Source: CAD feature listing. Evaluate the final solid. Frame: model axes, mm. Round coordinates to 2 decimals unless told otherwise and drop trailing zeros. Loops run counter-clockwise (first coordinate to the right, second up) from the corner with the lowest first, then second, coordinate; pieces in that order, holes last.
(1) Section D-D, the plane y = 15.5. Return the cut outline in (x, z).
(2) Section C-C, the plane z = -12. Return the cut outline in (x, y), plus the area to 3 significant figures.
(3) Section B-B, the plane y = -10. Return the cut outline in (x, z), plus the area to 3 significant figures.
(4) Material intervals for probe 1 along Y at (x, z) = (0, -24.5); probe 2 along Y at (x, z) = (0, -1.3), sorted ascending.
(5) Section A-A, the plane x = 0. Return the cut outline in (y, z).
(6) First-contact query: pin 1 Ø1 at (y, z) = (-12, -12.5) entering from +X; pin 2 Ø12 at (x, z) = (-2.5, -11.5) entering from -Y; pin 3 Ø2 at (x, z) = (-14, -4.5) entering from -Y. Flat tips, straight axial feed; report the tip coordinate or a pass-through.
(7) Mould query, pull axis Y, two halves, no side actions, for faces 1 (the flat face through (6, 20, -30)), 2 (the flat face through (-8, -11, -5)), 3 (the cylindrical face through (-2.343, -17.847, -18.311)), 4 (the cylindrical face through (-4.336, 19.524, -14.79)). Classes: pulls with the +Y half, pulls with the -Y half, needs draft (parallel to the pull), parting line crosses it, or undercut.
```python
from build123d import *

# Parameters (mm, degrees)
F0_R     = 20
F0_R_2   = 13.25
F1_DEPTH = 5
F2_R     = 20
F2_R_2   = 18
F3_DEPTH = 25
F4_R     = 30
F4_R_2   = 18
F5_DEPTH = 2


with BuildPart() as f1:
    # F0 (on Top) → F1 (new body)
    with BuildSketch(Plane.XY):
        Circle(F0_R)
        Circle(F0_R_2, mode=Mode.SUBTRACT)
    extrude(amount=-F1_DEPTH)

    # F2 (on face) → F3 (join)
    with BuildSketch(Plane(origin=(0, 0, -5), x_dir=(1, 0, 0), z_dir=(0, 0, -1))):
        Circle(F2_R)
        Circle(F2_R_2, mode=Mode.SUBTRACT)
    extrude(amount=F3_DEPTH)

    # F4 (on face) → F5 (join)
    with BuildSketch(Plane(origin=(0, 0, -30), x_dir=(1, 0, 0), z_dir=(0, 0, -1))):
        Circle(F4_R)
        Circle(F4_R_2, mode=Mode.SUBTRACT)
    extrude(amount=F5_DEPTH)


solid = f1.part
```
Output values:
1. outline: (-25.69, -32) - (-9.15, -32) - (-9.15, -5) - (9.15, -5) - (9.15, -32) - (25.69, -32) - (25.69, -30) - (12.64, -30) - (12.64, 0) - (-12.64, 0) - (-12.64, -30) - (-25.69, -30) - close
2. outline: circle Ø40 at (0, 0); hole circle Ø36 at (0, 0)
2. area: 239 mm2
3. outline: (-28.28, -32) - (-14.97, -32) - (-14.97, -5) - (-8.69, -5) - (-8.69, 0) - (-17.32, 0) - (-17.32, -30) - (-28.28, -30) - close; (8.69, -5) - (14.97, -5) - (14.97, -32) - (28.28, -32) - (28.28, -30) - (17.32, -30) - (17.32, 0) - (8.69, 0) - close
3. area: 257 mm2
4. probe 1: y = -20 to -18, 18 to 20
4. probe 2: y = -20 to -13.25, 13.25 to 20
5. outline: (-30, -32) - (-18, -32) - (-18, -5) - (-13.25, -5) - (-13.25, 0) - (-20, 0) - (-20, -30) - (-30, -30) - close; (13.25, -5) - (18, -5) - (18, -32) - (30, -32) - (30, -30) - (20, -30) - (20, 0) - (13.25, 0) - close
6. pin 1: stops at x = 16.36
6. pin 2: stops at y = -20
6. pin 3: stops at y = -15.2
7. face 1: needs draft
7. face 2: undercut
7. face 3: undercut
7. face 4: parting line crosses it
